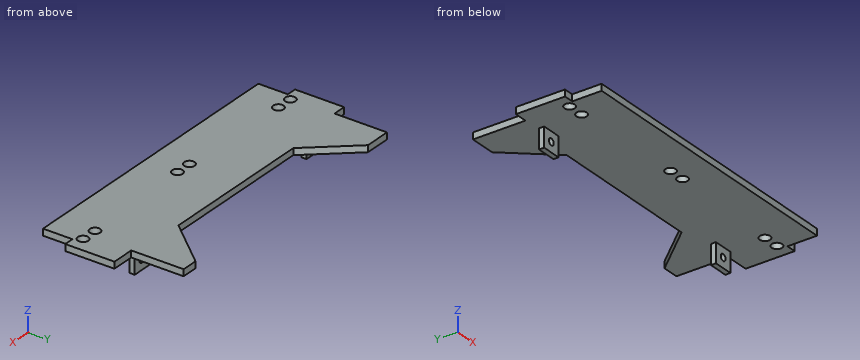
from build123d import *

# Parameters (mm, degrees)
SKETCH1_W           = 480
SKETCH1_H           = 200
BOSS_EXTRUDE1_DEPTH = 10
SKETCH2_W           = 30
SKETCH2_H           = 7.761380017
BOSS_EXTRUDE2_DEPTH = 30
SKETCH3_R           = 5
CUT_EXTRUDE1_DEPTH  = 30
SKETCH5_R           = 8
CUT_EXTRUDE2_DEPTH  = 30
SKETCH6_W           = 15
SKETCH6_H           = 45
SKETCH6_W_2         = 20
SKETCH6_H_2         = 80
SKETCH6_W_3         = 35
CUT_EXTRUDE3_DEPTH  = 10


with BuildPart() as part:
    # Sketch1 → Boss-Extrude1 (new body)
    with BuildSketch(Plane.XY):
        Rectangle(SKETCH1_W, SKETCH1_H)
    extrude(amount=BOSS_EXTRUDE1_DEPTH)

    # Sketch2 → Boss-Extrude2 (add)
    with BuildSketch(Plane(origin=(0, 0, 0), x_dir=(-1, 0, 0), z_dir=(0, 0, -1))):
        with Locations((-179.555, 13.880690009)):
            Rectangle(SKETCH2_W, SKETCH2_H)
        with Locations((179.555, 13.880690009)):
            Rectangle(SKETCH2_W, SKETCH2_H)
    extrude(amount=BOSS_EXTRUDE2_DEPTH)

    # Sketch3 → Cut-Extrude1 (cut)
    with BuildSketch(Plane(origin=(0, 17.761380017, 0), x_dir=(1, 0, 0), z_dir=(0, 1, 0))):
        with Locations((179.555, 15)):
            Circle(SKETCH3_R)
        with Locations((-179.555, 15)):
            Circle(SKETCH3_R)
    extrude(amount=-CUT_EXTRUDE1_DEPTH, mode=Mode.SUBTRACT)

    # Sketch5 → Cut-Extrude2 (cut)
    with BuildSketch(Plane.XY.offset(10)):
        with Locations((-12.5, -50)):
            Circle(SKETCH5_R)
        with Locations((-216.6, -45)):
            Circle(SKETCH5_R)
        with Locations((-191.6, -45)):
            Circle(SKETCH5_R)
        with Locations((12.5, -50)):
            Circle(SKETCH5_R)
        with Locations((191.6, -45)):
            Circle(SKETCH5_R)
        with Locations((216.6, -45)):
            Circle(SKETCH5_R)
        Polygon((140, 100), (90, 30), (-90, 30), (-140, 100), align=None)
    extrude(amount=-CUT_EXTRUDE2_DEPTH, mode=Mode.SUBTRACT)

    # Sketch6 → Cut-Extrude3 (cut)
    with BuildSketch(Plane(origin=(0, 0, 0), x_dir=(-1, 0, 0), z_dir=(0, 0, -1))):
        with Locations((-232.5, -77.5)):
            Rectangle(SKETCH6_W, SKETCH6_H)
        with Locations((232.5, -77.5)):
            Rectangle(SKETCH6_W, SKETCH6_H)
        with Locations((230, 60)):
            Rectangle(SKETCH6_W_2, SKETCH6_H_2)
        with Locations((-222.5, 60)):
            Rectangle(SKETCH6_W_3, SKETCH6_H_2)
        Polygon((140.207027179, 100), (180.207027179, 100), (120, 30), (90, 30), (114.970016322, 100), align=None)
        Polygon((-120, 30), (-90, 30), (-114.970016322, 100), (-140.207027179, 100), (-180.207027179, 100), align=None)
    extrude(amount=-CUT_EXTRUDE3_DEPTH, mode=Mode.SUBTRACT)


solid = part.part
Here's how the part is built. I have some questions about the finished solid (model axes, mm). Coordinates: 2 decimals unless noted, no trailing zeros. Loops run counter-clockwise (first coordinate to the right, second up) from the corner with the lowest first, then second, coordinate; pieces in that order, holes last.
1. Imagine slicing it at C-C, the plane y = 2.5. Please give me the cut outline in (x, z), and give its area (3 significant figures).
2. I need wall thicknesses on L1, parallel to X at y = 14, z = -15 (3 decimals); L2, parallel to Y at x = 207.5, z = 2.5; L3, parallel to Z at x = 182, y = -87.5. Which ranges of each line are inside material? Lowest first, please.
3. Imagine slicing it at A-A, the plane x = -12.5. Please give me the cut outline in (y, z).
4. For P1, Ø11, axis at x = -58.5, z = 4.5, coming from the +Y side; P2, Ø18.5, axis at x = -191.6, y = -45, coming from the -Z side; P3, Ø5, axis at x = 228.5, z = 7.5, coming from the +Y side, each with a flat end and sliding along its axis, tell me the tip position at first contact or that it passes through.
5. Imagine slicing it at B-B, the plane x = -90. Please give me the cut outline in (y, z), and give its area (3 significant figures).
Taken from the geometry:
1. outline: (-240, 0) - (240, 0) - (240, 10) - (-240, 10) - close
1. area: 4,800 mm2
2. L1: x = -194.555 to -184.555, -174.555 to -164.555, 164.555 to 174.555, 184.555 to 194.555
2. L2: y = -100 to 20
2. L3: z = 0 to 10
3. outline: (-100, 0) - (-58, 0) - (-58, 10) - (-100, 10) - close; (-42, 0) - (30, 0) - (30, 10) - (-42, 10) - close
4. P1: stops at y = 30
4. P2: stops at z = 0
4. P3: stops at y = 20
5. outline: (-100, 0) - (30, 0) - (30, 10) - (-100, 10) - close
5. area: 1,300 mm2
